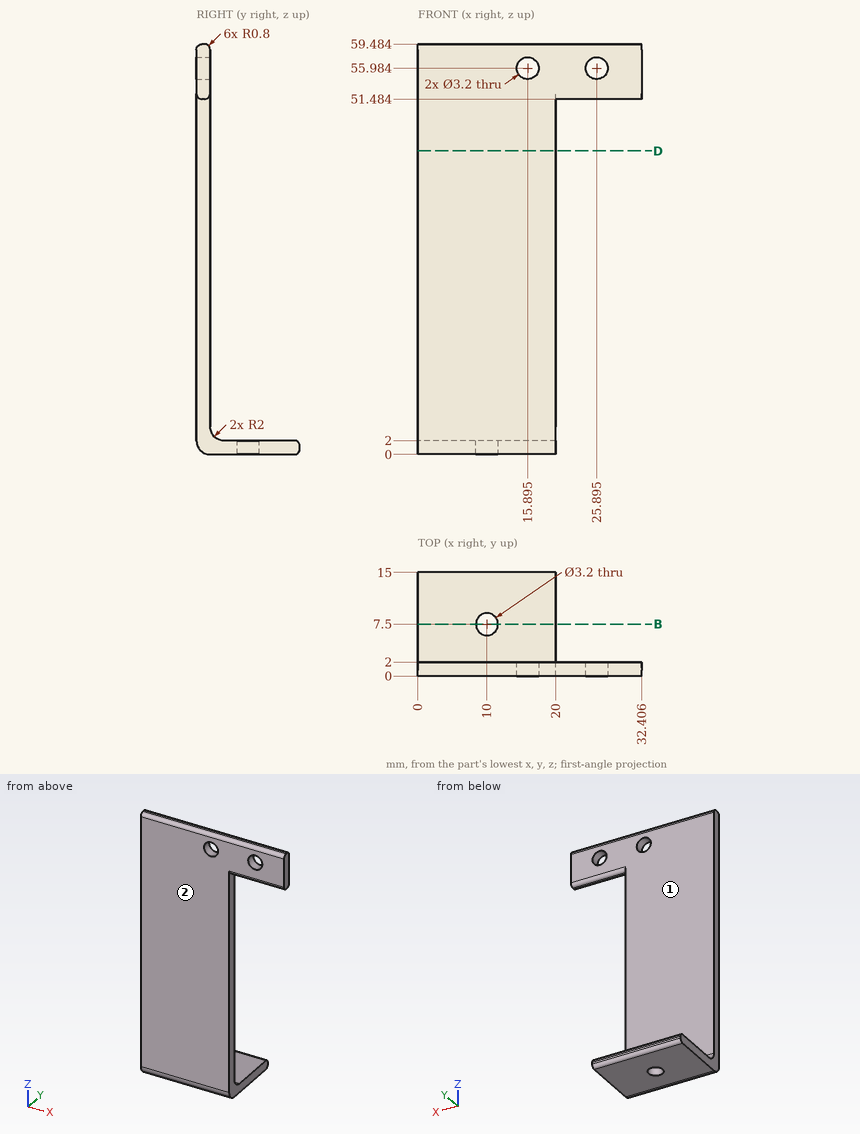
Verification items for this drawing (mm, ordinates from the low corner). A direction names the side the tool comes from. Coordinates: 2 decimals unless noted, no trailing zeros. Write each loop counter-clockwise with the first axis right and the second up, starting at its lowest first coordinate (ties: lowest second). Pieces come first, ordered by that corner, then holes. Notation, with made-up numbers: M -2,42.5 L 29,42.5 A19 cw 29,78.5 Z; hole C -12,-5.5 d1. An arc over 180 degrees is marked long. Answer as a JSON object with one key per item and string values. Group by question number.
(1) Cross-section at D-D, the plane z = 44. Record the cut outline in (x, y), and give its area (3 significant figures).
(2) Cross-section at B-B, the plane y = 7.5. Record the cut outline in (x, z), and give its area (3 significant figures).
(3) Gauge pin test, flat ends, axial feed: pin 1 (3 mm diameter, centred on x = 22.5, z = 51.5, fed in from +Y); pin 2 (8 mm diameter, centred on x = 29, y = 3, fed in from -Z). Record the tip position at first contact, or that the pin passes through.
(4) Tool access check on the marked faces 1 and 2. Record the directions out of +Z, -Z, +X, -X, +Y, -Y that give a thin tool (end or side, any length) a straight path to the whole face; none if there is none.
(5) Material ranges on line 1 (Y direction, x = 4.5, z = 34); line 2 (X direction, y = 1, z = 18), recorded low to high.
Reply:
{
 "1": {"outline": "M 0,0 L 20,0 L 20,2 L 0,2 Z", "area": "40.0 mm²"},
 "2": {"outline": "M 0,0 L 8.4,0 L 8.4,2 L 0,2 Z; M 11.6,0 L 20,0 L 20,2 L 11.6,2 Z", "area": "33.6 mm²"},
 "3": {"pin 1": "y = 2", "pin 2": "z = 51.48"},
 "4": {"face 1": "+Z, +X, -X, +Y", "face 2": "+Z, -Z, +X, -X, -Y"},
 "5": {"line 1": "0 to 2", "line 2": "0 to 20"}
}
